Source: three-view drawing plus pictorial views. Frame: mm from the lowest corner of the part. Coordinates: 2 decimals unless noted, no trailing zeros. Order: outer loops, then holes, each group sorted by start corner. A loop starts at its lowest first (then second) coordinate and runs counter-clockwise, first axis right, second up. Notation, with made-up numbers: (10.25, 19.25) -> (69.25, 19.25) arc R20 ccw to (69.25, 27.25) -> close; hole circle Ø1 at (-23, -24). An arc over 180 degrees is marked (long way). Use one line per item in the form item = value. Start each with the question number.
1) Section query A-A on x = 36. Output: boundary loops of the cut face in (y, z).
2) Ray query, line 1 along Z through (x, y) = (36, 0.85); line 2 along X through (y, z) = (1, 30.25); line 3 along Z through (x, y) = (7.5, 0.3). Return the intervals inside material, ascending.
3) Section query B-B on z = 30.25. Output: boundary loops of the cut face in (x, y), then the cut area to 3 significant figures.
4) Pin query (flat end, axial travel): pin 1 (1.6 mm diameter, centred on x = 36, z = 2.75, fed in from +Y). Return the tip coordinate at first contact, or that it passes through.
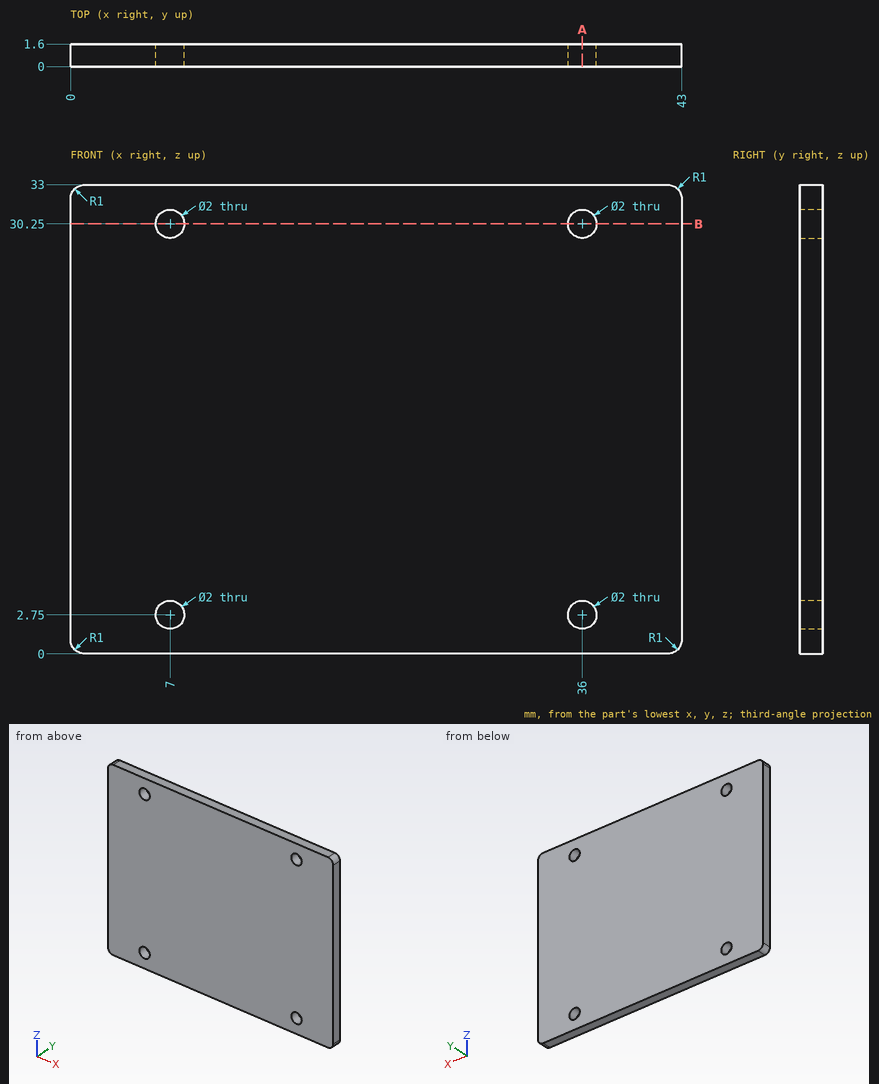
Answers below:
q1.outline = (0, 0) -> (1.6, 0) -> (1.6, 1.75) -> (0, 1.75) -> close; (0, 3.75) -> (1.6, 3.75) -> (1.6, 29.25) -> (0, 29.25) -> close; (0, 31.25) -> (1.6, 31.25) -> (1.6, 33) -> (0, 33) -> close
q2.line_1 = 0 to 1.75, 3.75 to 29.25, 31.25 to 33
q2.line_2 = 0 to 6, 8 to 35, 37 to 43
q2.line_3 = 0 to 1.88, 3.62 to 29.38, 31.12 to 33
q3.outline = (0, 0) -> (6, 0) -> (6, 1.6) -> (0, 1.6) -> close; (8, 0) -> (35, 0) -> (35, 1.6) -> (8, 1.6) -> close; (37, 0) -> (43, 0) -> (43, 1.6) -> (37, 1.6) -> close
q3.area = 62.4 mm^2
q4.pin_1 = through
